Verification items for the finished model (mm, model axes). Round coordinates to 2 decimals unless told otherwise and drop trailing zeros. Write each loop counter-clockwise with the first axis right and the second up, starting at its lowest first coordinate (ties: lowest second). Pieces come first, ordered by that corner, then holes. Notation, with made-up numbers: (88.5, 60.5) - (101.5, 60.5) arc R17 ccw to (101.5, 89.5) - close; hole circle Ø1 at (58, -37). An arc over 180 degrees is marked (long way). Answer as a JSON object with one key per item and string values. Group by question number.
1) Go/stop test with a flat-tipped pin: pin 1 Ø2.5 at (x, y) = (-8, 0) entering from -Z. Record where the tip stops, or that it passes through.
2) Section check C-C (y = 0). Enter the section's corners in (x, z), then the cut area to 3 significant figures.
3) Section check D-D (y = 8). Enter the section's corners in (x, z).
4) Section check B-B (z = 0.9). Enter the section's corners in (x, y), then the cut area to 3 significant figures.
5) Thickness scan on line 1 (Y direction, x = 0, z = 2.4); line 2 (X direction, y = -0.75, z = 4.2); line 3 (Y direction, x = -8, z = 2.05). Record the ranges inside material, lowest first.
6) Section check A-A (x = 0). Enter the section's corners in (y, z).
```python
from build123d import *

# Parameters (mm, degrees)
SZKIC1_R                    = 3
SZKIC1_R_2                  = 1.5
DODANIE_WYCI_GNI_CIE1_DEPTH = 5


with BuildPart() as part:
    # Szkic1 → Dodanie-wyciągnięcie1 (new body)
    with BuildSketch(Plane.XY):
        with BuildLine():
            Line((-50.67287635, 5.055665151), (-9.235111676, 10.570763761))
            ThreePointArc((-9.235111676, 10.570763761), (0, 11.182632843), (9.235111676, 10.570763761))
            Line((9.235111676, 10.570763761), (50.67287635, 5.055665151))
            ThreePointArc((50.67287635, 5.055665151), (55.100246338, 0), (50.67287635, -5.055665151))
            Line((50.67287635, -5.055665151), (9.235111676, -10.570763761))
            ThreePointArc((9.235111676, -10.570763761), (0, -11.182632843), (-9.235111676, -10.570763761))
            Line((-9.235111676, -10.570763761), (-50.67287635, -5.055665151))
            ThreePointArc((-50.67287635, -5.055665151), (-55.100246338, 0), (-50.67287635, 5.055665151))
        make_face()
        Circle(SZKIC1_R, mode=Mode.SUBTRACT)
        with Locations((0, 8)):
            Circle(SZKIC1_R_2, mode=Mode.SUBTRACT)
        with Locations((-8, 0)):
            Circle(SZKIC1_R_2, mode=Mode.SUBTRACT)
        with Locations((8, 0)):
            Circle(SZKIC1_R_2, mode=Mode.SUBTRACT)
        with Locations((0, -8)):
            Circle(SZKIC1_R_2, mode=Mode.SUBTRACT)
        with Locations((-50, 0)):
            Circle(SZKIC1_R, mode=Mode.SUBTRACT)
        with Locations((50, 0)):
            Circle(SZKIC1_R, mode=Mode.SUBTRACT)
    extrude(amount=DODANIE_WYCI_GNI_CIE1_DEPTH)


solid = part.part
```
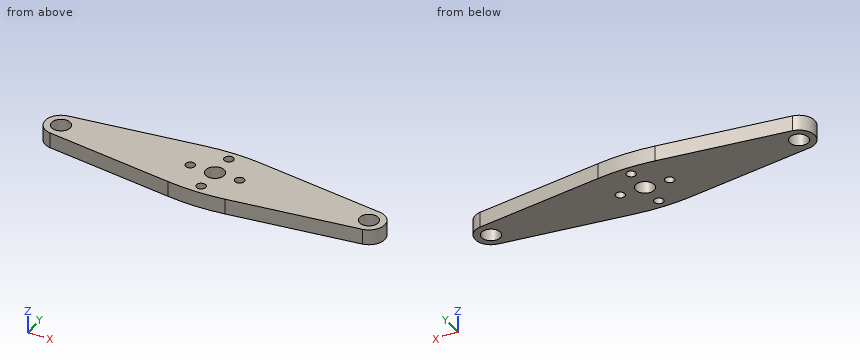
Returned:
{
 "1": {"pin 1": "through"},
 "2": {"outline": "(-55.1, 0) - (-53, 0) - (-53, 5) - (-55.1, 5) - close; (-47, 0) - (-9.5, 0) - (-9.5, 5) - (-47, 5) - close; (-6.5, 0) - (-3, 0) - (-3, 5) - (-6.5, 5) - close; (3, 0) - (6.5, 0) - (6.5, 5) - (3, 5) - close; (9.5, 0) - (47, 0) - (47, 5) - (9.5, 5) - close; (53, 0) - (55.1, 0) - (55.1, 5) - (53, 5) - close", "area": "431 mm2"},
 "3": {"outline": "(-28.55, 0) - (-1.5, 0) - (-1.5, 5) - (-28.55, 5) - close; (1.5, 0) - (28.55, 0) - (28.55, 5) - (1.5, 5) - close"},
 "4": {"outline": "(-50.67, -5.06) - (-9.24, -10.57) arc R70 ccw to (9.24, -10.57) - (50.67, -5.06) arc R5.1 ccw to (50.67, 5.06) - (9.24, 10.57) arc R70 ccw to (-9.24, 10.57) - (-50.67, 5.06) arc R5.1 ccw to start; hole circle Ø6 at (-50, 0); hole circle Ø3 at (-8, 0); hole circle Ø6 at (0, 0); hole circle Ø3 at (0, -8); hole circle Ø3 at (0, 8); hole circle Ø3 at (8, 0); hole circle Ø6 at (50, 0)", "area": "1,660 mm2"},
 "5": {"line 1": "-11.18 to -9.5, -6.5 to -3, 3 to 6.5, 9.5 to 11.18", "line 2": "-55.04 to -52.9, -47.1 to -9.3, -6.7 to -2.9, 2.9 to 6.7, 9.3 to 47.1, 52.9 to 55.04", "line 3": "-10.72 to -1.5, 1.5 to 10.72"},
 "6": {"outline": "(-11.18, 0) - (-9.5, 0) - (-9.5, 5) - (-11.18, 5) - close; (-6.5, 0) - (-3, 0) - (-3, 5) - (-6.5, 5) - close; (3, 0) - (6.5, 0) - (6.5, 5) - (3, 5) - close; (9.5, 0) - (11.18, 0) - (11.18, 5) - (9.5, 5) - close"}
}
